from build123d import *

# Parameters (mm, degrees)
SKETCH_1_R           = 30
EXTRUDE_1_DEPTH      = 40
EXTRUDE_2_DEPTH      = 20
SKETCH_2_R           = 20
SKETCH_2_R_2         = 10
EXTRUDE_3_DEPTH      = 20
CUT_EXTRUDE_1_DEPTH  = 20
EXTRUDE_4_REACH      = 174.452
EXTRUDE_4_END_RADIUS = 30
SKETCH_3_R           = 3.75
CUT_EXTRUDE_2_REACH  = 174.452
SKETCH_3_2_R         = 3.75


with BuildPart() as part:
    # 草图1 → 凸台-拉伸1 (new body)
    with BuildSketch(Plane.XY):
        Circle(SKETCH_1_R)
        with BuildLine():
            ThreePointArc((-4, 14.456832295), (0, -15), (4, 14.456832295))
            Line((4, 14.456832295), (4, 20))
            Line((4, 20), (-4, 20))
            Line((-4, 20), (-4, 14.456832295))
        make_face(mode=Mode.SUBTRACT)
    extrude(amount=EXTRUDE_1_DEPTH)

    # 草图1<3> → 凸台-拉伸2 (add)
    with BuildSketch(Plane.XY):
        with BuildLine():
            Line((-69.996355211, 0.714322908), (-106.066017178, -35.355339059))
            Line((-106.066017178, -35.355339059), (-91.923881554, -49.497474683))
            Line((-91.923881554, -49.497474683), (-75.985459186, -33.559052315))
            ThreePointArc((-75.985459186, -33.559052315), (-46.930334751, -19.312906561), (-15.236295048, -25.842896765))
            ThreePointArc((-15.236295048, -25.842896765), (-28.981985351, 7.748840242), (-0.306138389, 29.998437947))
            ThreePointArc((-0.306138389, 29.998437947), (-38.024919972, 22.195136051), (-69.996355211, 0.714322908))
        make_face()
    extrude(amount=EXTRUDE_2_DEPTH)

    # 草图2 → 凸台-拉伸3 (add)
    with BuildSketch(Plane(origin=(-21.213203436, 21.213203436, 0), x_dir=(0, 0, -1), z_dir=(0.7071067811865452, -0.7071067811865498, 0))):
        with Locations((-10, -100)):
            Circle(SKETCH_2_R)
        with Locations((-10, -100)):
            Circle(SKETCH_2_R_2, mode=Mode.SUBTRACT)
    extrude(amount=-EXTRUDE_3_DEPTH)

    # 草图2<3> → 切除-拉伸1 (cut)
    with BuildSketch(Plane(origin=(-21.213203436, 21.213203436, 0), x_dir=(0, 0, -1), z_dir=(0.7071067811865452, -0.7071067811865498, 0))):
        with BuildLine():
            Line((-20, -100), (0, -100))
            ThreePointArc((0, -100), (-10, -90), (-20, -100))
        make_face()
        with BuildLine():
            ThreePointArc((-20, -100), (-10, -110), (0, -100))
            Line((0, -100), (-20, -100))
        make_face()
    extrude(amount=-CUT_EXTRUDE_1_DEPTH, mode=Mode.SUBTRACT)

    # 凸台-拉伸4: up to this cylinder (the profile starts outside it)
    extrude_4_end = Plane(origin=(0, 0, 30.224226), z_dir=(0, 0, -1)) * Cylinder(EXTRUDE_4_END_RADIUS, 409.904, mode=Mode.PRIVATE)
    # 草图3 → 凸台-拉伸4 (add, up to the surface)
    with BuildSketch(Plane(origin=(35, 0, 0), x_dir=(0, 0, -1), z_dir=(1, 0, 0)), mode=Mode.PRIVATE) as extrude_4_sk1:
        with BuildLine():
            Line((-25, 7.5), (-40, 7.5))
            Line((-40, 7.5), (-40, -7.5))
            Line((-40, -7.5), (-25, -7.5))
            ThreePointArc((-25, -7.5), (-17.5, 0), (-25, 7.5))
        make_face()
        with Locations((-25, 0)):
            Circle(SKETCH_3_R, mode=Mode.SUBTRACT)
    extrude_4_tool1 = extrude(extrude_4_sk1.sketch, amount=-EXTRUDE_4_REACH, mode=Mode.PRIVATE) - extrude_4_end
    add(extrude_4_tool1.solids().sort_by_distance((35, 0, 30.224226))[0])

    # 草图3<2> → 切除-拉伸2 (cut, up to next)
    with BuildSketch(Plane(origin=(35, 0, 0), x_dir=(0, 0, -1), z_dir=(1, 0, 0)), mode=Mode.PRIVATE) as cut_extrude_2_sk1:
        with Locations((-25, 0)):
            Circle(SKETCH_3_2_R)
    cut_extrude_2_tool1 = extrude(cut_extrude_2_sk1.sketch, amount=-CUT_EXTRUDE_2_REACH, mode=Mode.PRIVATE) & part.part
    add(cut_extrude_2_tool1.solids().sort_by_distance((35, 0, 25))[0], mode=Mode.SUBTRACT)


solid = part.part
The model under review builds one solid part; all positions refer to its coordinate system, in mm. A direction names the side the tool comes from. Round coordinates to 2 decimals unless told otherwise and drop trailing zeros. Order: outer loops, then holes, each group sorted by start corner. A loop starts at its lowest first (then second) coordinate and runs counter-clockwise, first axis right, second up. Notation, with made-up numbers: (66, 68.5) -> (102, 68.5) arc R25 ccw to (102, 81.5) -> close; hole circle Ø7 at (-12.5, -32). An arc over 180 degrees is marked (long way). Write item = value, one per line. Start each with the question number.
Item 1: Consider section C-C on x = -12. Write out the cut boundary in (y, z), plus the area to 3 significant figures.
Item 2: For line 1 along Z through (x, y) = (25, 0); line 2 along Z through (x, y) = (31.3, 0); line 3 along Y through (x, z) = (32, 25), list the stretches that pass through material, from the lowest coordinate up.
Item 3: For faces 1 (the face through (32, -7.5, 33)), 2 (the face through (32, 7.5, 32)), 3 (the face through (0, 20, 20)), 4 (the face through (-113.029, -56.658, 10.733)), 5 (the face through (32.07, -0.16, 17.5)), list the 3-axis set-ups (+Z, -Z, +X, -X, +Y, -Y) from which the entire face can be reached by the end or side of a thin tool; tool diameter is ignored.
Item 4: Consider section A-A on z = 10. Write out the cut boundary in (x, y), plus the area to 3 significant figures.
Item 5: Mouldability with a two-part tool opening along Y and no side actions: class faces 6 (the face through (27.712, -11.49, 24.164)), 7 (the face through (-4, 17, 20)), 8 (the face through (35, 0, 31)), 9 (the face through (4, 17, 20)) as released by +Y, released by -Y, zero draft, split by the parting line, or undercut.
Item 6: Clearance check with flat-ended pins moving along their axes: pin 1 Ø6.5 at (x, z) = (32.5, 32) entering from +Y; pin 2 Ø8 at (y, z) = (-12.5, 19) entering from +X; pin 3 Ø5 at (x, z) = (-104, 26) entering from -Y. State where each tip first meets the part, or that it passes through.
Item 7: Consider section B-B on y = -5.5. Write out the cut boundary in (x, z), plus the area to 3 significant figures.
Item 8: Consider section D-D on z = 33. Write out the cut boundary in (x, y), plus the area to 3 significant figures.
Conclusion:
q1.outline = (-27.5, 0) -> (-9, 0) -> (-9, 40) -> (-27.5, 40) -> close; (9, 0) -> (29.19, 0) -> (29.19, 20) -> (27.5, 20) -> (27.5, 40) -> (9, 40) -> close
q1.area = 1,510 mm2
q2.line_1 = 0 to 21.25, 28.75 to 40
q2.line_2 = 17.5 to 21.25, 28.75 to 40
q2.line_3 = -7.5 to -3.75, 3.75 to 7.5
q3.face_1 = +Z, -Z, +X, -Y
q3.face_2 = +Z, -Z, +X, +Y
q3.face_3 = +Z, -Z
q3.face_4 = none
q3.face_5 = -Z, +X
q4.outline = (-120.21, -49.5) -> (-106.07, -63.64) -> (-98.99, -56.57) -> (-113.14, -42.43) -> close; (-98.99, -28.28) -> (-84.85, -42.43) -> (-75.99, -33.56) arc R50 cw to (-15.24, -25.84) arc R30 ccw (long way) to (-0.31, 30) arc R100 ccw to (-70, 0.71) -> close; hole (-4, 14.46) arc R15 ccw (long way) to (4, 14.46) -> (4, 20) -> (-4, 20) -> close
q4.area = 4,560 mm2
q5.face_6 = split by the parting line
q5.face_7 = undercut
q5.face_8 = zero draft
q5.face_9 = undercut
q6.pin_1 = 7.5
q6.pin_2 = 28.77
q6.pin_3 = -59.12
q7.outline = (-76.21, 0) -> (-13.96, 0) -> (-13.96, 40) -> (-29.49, 40) -> (-29.49, 20) -> (-76.21, 20) -> close; (13.96, 0) -> (29.49, 0) -> (29.49, 19.9) -> (35, 19.9) -> (35, 40) -> (13.96, 40) -> close
q7.area = 2,290 mm2
q8.outline = (29.05, -7.5) -> (35, -7.5) -> (35, 7.5) -> (29.05, 7.5) arc R30 ccw (long way) to start; hole (-4, 14.46) arc R15 ccw (long way) to (4, 14.46) -> (4, 20) -> (-4, 20) -> close
q8.area = 2,160 mm2
